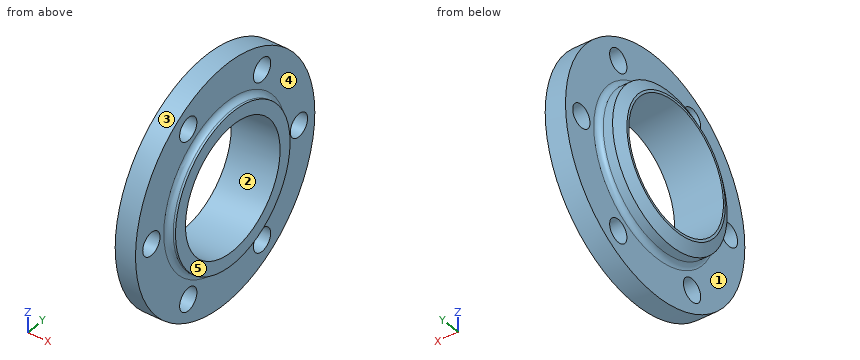
```python
from build123d import *

# Parameters (mm, degrees)
F1_W          = 9.5356404781
F1_H          = 20.2632434666
F3_R          = 2.54
F4_R          = 2.54
F5_SIZE2      = 5.08
F5_SIZE       = 2.9329393675
F6_R          = 5.4033891953
F7_DEPTH      = 25.4
F7_DEPTH_BACK = 25.4
F8_DEPTH      = 25.4
F8_DEPTH_BACK = 25.4


with BuildPart() as f2:
    # F1 (on Top) → F2 (revolve)
    with BuildSketch(Plane.XY):
        with Locations((44.84731704, 46.0392739624)):
            Rectangle(F1_W, F1_H)
        Polygon((49.615137279, 35.9076522291), (40.0794968009, 35.9076522291), (30.2458684891, 35.9076522291), (30.2458684891, 29.6498890966), (53.1910024583, 29.6498890966), (53.1910024583, 35.9076522291), align=None)
    revolve(axis=Axis((0.2979896963, 0, 0), (1, 0, 0)))

    # F3
    f3_edges = [f2.edges().sort_by_distance(p)[0] for p in [
        (49.615137, -35.907652, 0),
    ]]
    fillet(f3_edges, radius=F3_R)

    # F4
    f4_edges = [f2.edges().sort_by_distance(p)[0] for p in [
        (40.079497, -35.907652, 0),
    ]]
    fillet(f4_edges, radius=F4_R)

    # F5
    f5_edges = [f2.edges().sort_by_distance(p)[0] for p in [
        (30.245868, -35.907652, 0),
    ]]
    f5_side = f2.faces().sort_by_distance((33.892683, -35.907652, 0))[0]
    chamfer(f5_edges, length=F5_SIZE, length2=F5_SIZE2, reference=f5_side)

    # F6 (on face) → F7 (cut, two sides)
    with BuildSketch(Plane(origin=(40.0794968009, 0, 0), x_dir=(0, -1, 0), z_dir=(-1, 0, 0))) as f7_sk:
        with Locations((-46.2401774935, 0)):
            Circle(F6_R)
    extrude(amount=F7_DEPTH, mode=Mode.SUBTRACT)
    extrude(f7_sk.sketch, amount=-F7_DEPTH_BACK, mode=Mode.SUBTRACT)

    # F6 (on face) → F8 (cut, two sides)
    with BuildSketch(Plane(origin=(40.0794968009, 0, 0), x_dir=(0, -1, 0), z_dir=(-1, 0, 0))) as f8_sk:
        with Locations((-46.2401774935, 0)):
            Circle(F6_R)
        with Locations((-23.1200887467, -40.0451683849)):
            Circle(F6_R)
        with Locations((23.1200887467, -40.0451683849)):
            Circle(F6_R)
        with Locations((46.2401774935, 0)):
            Circle(F6_R)
        with Locations((23.1200887467, 40.0451683849)):
            Circle(F6_R)
        with Locations((-23.1200887467, 40.0451683849)):
            Circle(F6_R)
    extrude(amount=-F8_DEPTH, mode=Mode.SUBTRACT)
    extrude(f8_sk.sketch, amount=F8_DEPTH_BACK, mode=Mode.SUBTRACT)


solid = f2.part
```
For this review, take the finished solid that the model builds, in its own axes (mm). Face numbers are marked on the shaded views. A direction names the side the tool comes from. Round coordinates to 2 decimals unless told otherwise and drop trailing zeros. Write each loop counter-clockwise with the first axis right and the second up, starting at its lowest first coordinate (ties: lowest second). Pieces come first, ordered by that corner, then holes. Notation, with made-up numbers: (-6, 63) -> (27, 63) arc R18 ccw to (27, 78) -> close; hole circle Ø1 at (78.25, 33). An arc over 180 degrees is marked (long way). One line per question, with ' | ' between items. Start each with the question number.
(1) Add section A-A, the plane y = 0. Write out the cut boundary in (x, z), plus the area to 3 significant figures.
(2) Add section D-D, the plane y = 48.5. Write out the cut boundary in (x, z), plus the area to 3 significant figures.
(3) Add section B-B, the plane z = 0. Give the number of separate pieces and of enclosed holes in the cut face, plus the area to 3 significant figures.
(4) Mouldability with a two-part tool opening along Y and no side actions: class the marked faces 1, 2 and 3 as released by +Y, released by -Y, zero draft, split by the parting line, or undercut.
(5) For line 1 along Z through (x, y) = (37.25, 0); line 2 along Y through (x, z) = (45.25, -43.5); line 3 along X through (y, z) = (19.5, -46), list the stretches that pass through material, from the lowest coordinate up. Write a range as from..to.
(6) Add section C-C, the plane y = -43.5. Write out the cut boundary in (x, z).
(7) Tool access review of the marked faces 4 and 5: name each direction out of +Z, -Z, +X, -X, +Y, -Y from which nothing blocks a thin tool from reaching the whole face with its end or side.
(8) Insertion check: P1, Ø17.5, axis at y = 23.12, z = -40.05, coming from the -X side; P2, Ø8.5, axis at y = 46.24, z = 0, coming from the -X side; P3, Ø12, axis at x = 41, y = 43, coming from the +Z side; P4, Ø1, axis at y = 13.5, z = -35, coming from the +X side. Each pin has a flat end and moves straight along its axis. Give the tip position at first contact, or say it passes through.
Answer list:
1) outline: (30.25, -30.83) -> (33.18, -35.91) -> (37.54, -35.91) arc R2.54 cw to (40.08, -38.45) -> (40.08, -56.17) -> (49.62, -56.17) -> (49.62, -38.45) arc R2.54 cw to (52.16, -35.91) -> (53.19, -35.91) -> (53.19, -29.65) -> (30.25, -29.65) -> close; (30.25, 29.65) -> (53.19, 29.65) -> (53.19, 35.91) -> (52.16, 35.91) arc R2.54 cw to (49.62, 38.45) -> (49.62, 56.17) -> (40.08, 56.17) -> (40.08, 38.45) arc R2.54 cw to (37.54, 35.91) -> (33.18, 35.91) -> (30.25, 30.83) -> close | area: 664 mm²
2) outline: (40.08, -28.34) -> (49.62, -28.34) -> (49.62, -4.91) -> (40.08, -4.91) -> close; (40.08, 4.91) -> (49.62, 4.91) -> (49.62, 28.34) -> (40.08, 28.34) -> close | area: 447 mm²
3) separate pieces: 4 | enclosed holes: 0 | area: 458 mm²
4) face 1: zero draft | face 2: undercut | face 3: split by the parting line
5) line 1: -35.91..-29.65, 29.65..35.91 | line 2: -35.54..-27.27, -18.97..18.97, 27.27..35.54 | line 3: 40.08..49.62
6) outline: (40.08, -35.54) -> (49.62, -35.54) -> (49.62, -4.66) -> (40.08, -4.66) -> close; (40.08, 4.66) -> (49.62, 4.66) -> (49.62, 35.54) -> (40.08, 35.54) -> close
7) face 4: +X | face 5: +Z, -Z, +X, +Y, -Y
8) P1: x = 39.89 | P2: through | P3: z = 42.26 | P4: x = 50.06
